Autodesk Fusion 360 part; units mm, degrees
sketch "Sketch1" plane through (0, 0, 0) normal (0, 0, 1) x (1, 0, 0) in component "Shaft"
  circle A0 centre (0, 0) radius 7
  dimension "d4" = 14
extrude "Extrude1" add sketch "Sketch1" along normal blind 50 in component "Shaft"
sketch "Sketch2" plane through (0, 0, 0) normal (0, 0, 1) x (1, 0, 0) in component "Shaft"
  circle A0 centre (0, 0) radius 2.6
  line L0 (1.7, 2.6) -> (-1.7, 2.6)
  line L1 (-1.7, 2.6) -> (-1.7, -2.6)
  line L2 (-1.7, -2.6) -> (1.7, -2.6)
  line L3 (1.7, -2.6) -> (1.7, 2.6)
  line L4 (1.7, 2.6) -> (-1.7, -2.6) construction
  line L5 (-1.7, 2.6) -> (1.7, -2.6) construction
  dimension "d8" = 5.2
  dimension "d9" = 3.4
  dimension "d10" = 5.2
extrude "Extrude2" cut sketch "Sketch2" along normal blind 6 contours A0 L1 L3 in component "Shaft"
sketch "Sketch3" plane through (0, 0, 0) normal (0, 1, 0) x (1, 0, 0) in component "Shaft"
  line L0 (-7, -50) -> (7, -50)
  line L1 (0, 0) -> (0, -50) construction
  circle A0 centre (0, -25) radius 1.125
  dimension "d15" = 50
  dimension "d16" = 2.25
extrude "Extrude3" cut sketch "Sketch3" along normal blind 7 and the other way blind 7 in component "Shaft"
component "Shaft" placed x (1, 0, 0) y (0, 1, 0) z (0, 0, 1) at (0, 0, 0)
equation "shaftOuterDiameter = 14 mm"
equation "shaftInnerDiameter = 5.2 mm"
equation "shaftInnerSmallDiameter = 3.4 mm"
equation "d4 = shaftOuterDiameter"
equation "shaftHeight = 50 mm"
equation "d6 = shaftHeight"
equation "d8 = shaftInnerDiameter"
equation "d9 = shaftInnerSmallDiameter"
equation "d10 = shaftInnerDiameter"
equation "shaftSmallDepth = 6 mm"
equation "d12 = shaftSmallDepth"
equation "shaftDrillHole = 2.25 mm"
equation "d15 = shaftHeight"
equation "d16 = shaftDrillHole"
equation "d17 = shaftOuterDiameter / 2"
equation "d19 = shaftOuterDiameter / 2"
Model file for the job. Use its own axes, mm. A direction names the side the tool comes from. Coordinates: 2 decimals unless noted, no trailing zeros. Loops run counter-clockwise (first coordinate to the right, second up) from the corner with the lowest first, then second, coordinate; pieces in that order, holes last. Notation, with made-up numbers: M -27,47 L -17,47 A17 cw -17,70 Z; hole C 0.5,-9.75 d9. An arc over 180 degrees is marked long. Use CSV: the item, a comma, the result in double quotes. Start each with the question number.
1. Band-saw the part on A-A, the plane x = 0. List the corners of the cut face in (y, z) (3 decimals), then the cut area to 3 significant figures.
2. Band-saw the part on B-B, the plane y = 0. List the corners of the cut face in (x, z) (3 decimals), then the cut area to 3 significant figures.
3. Flat gauge pins, fed straight in: pin 1 (1.5 mm diameter, centred on y = -4.5, z = 14, fed in from +X); pin 2 (1 mm diameter, centred on x = 5, z = 34.5, fed in from -Y); pin 3 (2 mm diameter, centred on y = -4.5, z = 45, fed in from -X); pin 4 (4.5 mm diameter, centred on y = 1, z = 1.5, fed in from +X). Where does each tip first touch, or does it go through?
4. Band-saw the part on D-D, the plane x = -5.5. List the corners of the cut face in (y, z), then the cut area to 3 significant figures.
5. Two-plate mould, pull along Y, no slides. Class faces 1 (the cylindrical face through (-0.146, 0.098, 23.885)), 2 (the cylindrical face through (-1.517, 6.834, 24.65)), 3 (the flat face through (-1.7, 0, 3)): pulls with the +Y half, pulls with the -Y half, needs draft (parallel to the pull), parting line crosses it, or undercut.
6. Band-saw the part on C-C, the plane z = 29.5. List the corners of the cut face in (x, y), then the cut area to 3 significant figures.
7. Tool access for faces 4 (the flat face through (1.7, 0, 3)), 5 (the flat face through (0, 0, 50)): list every direction of +Z, -Z, +X, -X, +Y, -Y with a clear straight run to the whole face (end or side of a thin tool).
8. Probe probe 1 along Z at (x, y) = (0, 4) (3 decimals); probe 2 along X at (y, z) = (0.25, 25) (3 decimals); probe 3 along Z at (x, y) = (0, -1.5) (3 decimals). List the from-to ranges inside material, lowest first. Write a range as [from, to].
Entries:
1,outline,"M -7,0 L -2.6,0 L -2.6,6 L 2.6,6 L 2.6,0 L 7,0 L 7,23.875 L -7,23.875 Z; M -7,26.125 L 7,26.125 L 7,50 L -7,50 Z"
1,area,"637 mm2"
2,outline,"M -7,0 L -1.7,0 L -1.7,6 L 1.7,6 L 1.7,0 L 7,0 L 7,50 L -7,50 Z; hole C 0,25 d2.25"
2,area,"676 mm2"
3,pin 1,"stops at x = 5.91"
3,pin 2,"stops at y = -5.36"
3,pin 3,"stops at x = -6.06"
3,pin 4,"stops at x = 7"
4,outline,"M -4.33,0 L 4.33,0 L 4.33,50 L -4.33,50 Z"
4,area,"433 mm2"
5,face 1,"needs draft"
5,face 2,"parting line crosses it"
5,face 3,"undercut"
6,outline,"C 0,0 d14"
6,area,"154 mm2"
7,face 4,"-Z"
7,face 5,"+Z, +X, -X, +Y, -Y"
8,probe 1,"z = [0, 23.875], [26.125, 50]"
8,probe 2,"x = [-6.996, -1.125], [1.125, 6.996]"
8,probe 3,"z = [6, 23.875], [26.125, 50]"
